The model under review builds one solid part; all positions refer to its coordinate system, in mm. Face numbers are marked on the shaded views. Round coordinates to 2 decimals unless told otherwise and drop trailing zeros. Loops run counter-clockwise (first coordinate to the right, second up) from the corner with the lowest first, then second, coordinate; pieces in that order, holes last. Notation, with made-up numbers: (-22, -4) -> (14, -4) arc R21 cw to (14, 25) -> close; hole circle Ø9 at (-1.75, 80.5). An arc over 180 degrees is marked (long way). Use a Markdown table: item, result. Add a question column.
1) Consider section B-B on z = 0. Give the boundary of the cut face in (x, y).
2) Mouldability with a two-part tool opening along Z and no side actions: class the marked faces 1, 2, 3 and 4 as released by +Z, released by -Z, zero draft, split by the parting line, or undercut.
3) Consider section A-A on y = 8.25. Give the boundary of the cut face in (x, z).
4) Consider section C-C on x = 0. Give the boundary of the cut face in (y, z), plus the area to 3 significant figures.
5) Wall thickness on probe 1 along Z at (x, y) = (5, 5.5); probe 2 along Z at (x, y) = (6.5, 20.25); probe 3 along Y at (x, z) = (-9, -6.5): over which ranges is each line inside the solid? List them lowest first.
6) Insertion check: pin 1 (8 mm diameter, centred on x = -6.5, y = 8, fed in from +Z); pin 2 (16 mm diameter, centred on y = 18, z = 4, fed in from -X); pin 3 (5 mm diameter, centred on x = -12.5, y = 20.5, fed in from -Z). Each pin has a flat end and moves straight along its axis. Give the tip position at first contact, or say it passes through.
7) Consider section D-D on x = 12. Give the boundary of the cut face in (y, z), plus the area to 3 significant figures.
from build123d import *

# Parameters (mm, degrees)
SKETCH1_R           = 15
SKETCH1_W           = 20
SKETCH1_H           = 20
BOSS_EXTRUDE1_DEPTH = 27.1
SKETCH2_R           = 16
BOSS_EXTRUDE2_DEPTH = 1.5
BOSS_EXTRUDE4_START = -27.1
SKETCH3_R           = 15.15
SKETCH3_R_2         = 15
SKETCH3_W           = 20
SKETCH3_H           = 20
BOSS_EXTRUDE4_DEPTH = 27.1
CUT_EXTRUDE1_START  = -1.5
SKETCH4_R           = 15.15
CUT_EXTRUDE1_DEPTH  = 1.5


with BuildPart() as part:
    # Sketch1 → Boss-Extrude1 (new body)
    with BuildSketch(Plane(origin=(0, 0, 0), x_dir=(1, 0, 0), z_dir=(0, 1, 0))):
        with Locations(Location((0, 0, 0), (0, 0, 90))):
            Circle(SKETCH1_R)
        Rectangle(SKETCH1_W, SKETCH1_H, mode=Mode.SUBTRACT)
    extrude(amount=BOSS_EXTRUDE1_DEPTH)

    # Sketch2 → Boss-Extrude2 (add)
    with BuildSketch(Plane.XZ):
        with Locations(Location((0, 0, 0), (0, 0, 270))):
            Circle(SKETCH2_R)
    extrude(amount=BOSS_EXTRUDE2_DEPTH)

    # Sketch3 → Boss-Extrude4 (add)
    # profile 1 of 2: a face of its own
    with BuildSketch(Plane(origin=(0, 27.1, 0), x_dir=(1, 0, 0), z_dir=(0, 1, 0)).offset(BOSS_EXTRUDE4_START)):
        with Locations(Location((0, 0, 0), (0, 0, 270))):
            Circle(SKETCH3_R)
        Circle(SKETCH3_R_2, mode=Mode.SUBTRACT)
    # profile 2 of 2: a face of its own
    with BuildSketch(Plane(origin=(0, 27.1, 0), x_dir=(1, 0, 0), z_dir=(0, 1, 0)).offset(BOSS_EXTRUDE4_START)):
        Circle(SKETCH3_R_2)
        Rectangle(SKETCH3_W, SKETCH3_H, mode=Mode.SUBTRACT)
    extrude(amount=BOSS_EXTRUDE4_DEPTH)

    # Sketch4 → Cut-Extrude1 (cut)
    with BuildSketch(Plane(origin=(0, 27.1, 0), x_dir=(1, 0, 0), z_dir=(0, 1, 0)).offset(CUT_EXTRUDE1_START)):
        with Locations(Location((0, 0, 0), (0, 0, 270))):
            Circle(SKETCH4_R)
    extrude(amount=CUT_EXTRUDE1_DEPTH, mode=Mode.SUBTRACT)


solid = part.part
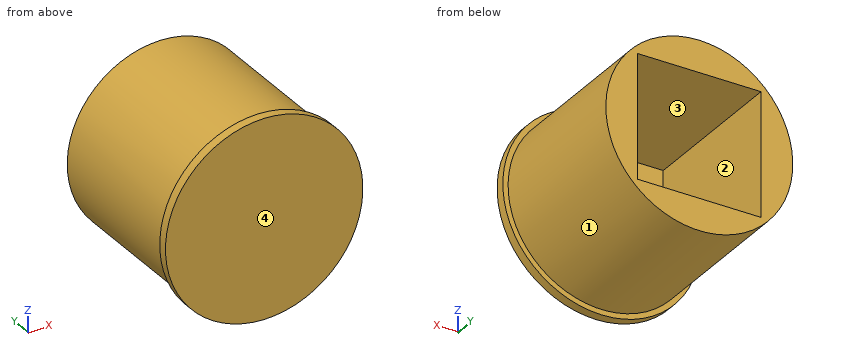
Result set:
| question | item | result |
|---|---|---|
| 1 | outline | (-16, -1.5) -> (16, -1.5) -> (16, 0) -> (15.15, 0) -> (15.15, 25.6) -> (10, 25.6) -> (10, 0) -> (-10, 0) -> (-10, 25.6) -> (-15.15, 25.6) -> (-15.15, 0) -> (-16, 0) -> close |
| 2 | face 1 | split by the parting line |
| 2 | face 2 | undercut |
| 2 | face 3 | undercut |
| 2 | face 4 | zero draft |
| 3 | outline | circle Ø30.3 at (0, 0); hole (-10, -10) -> (10, -10) -> (10, 10) -> (-10, 10) -> close |
| 4 | outline | (-1.5, -16) -> (0, -16) -> (0, -15.15) -> (25.6, -15.15) -> (25.6, -10) -> (0, -10) -> (0, 10) -> (25.6, 10) -> (25.6, 15.15) -> (0, 15.15) -> (0, 16) -> (-1.5, 16) -> close |
| 4 | area | 312 mm2 |
| 5 | probe 1 | -14.3 to -10, 10 to 14.3 |
| 5 | probe 2 | -13.68 to -10, 10 to 13.68 |
| 5 | probe 3 | -1.5 to 0 |
| 6 | pin 1 | z = 14.94 |
| 6 | pin 2 | x = -15.15 |
| 6 | pin 3 | z = -11.38 |
| 7 | outline | (-1.5, -10.58) -> (0, -10.58) -> (0, -9.25) -> (25.6, -9.25) -> (25.6, 9.25) -> (0, 9.25) -> (0, 10.58) -> (-1.5, 10.58) -> close |
| 7 | area | 505 mm2 |
